Input: part model. Units: mm. Frame: model coordinates. A direction names the side the tool comes from. Give positions to 0.01 mm unless a question says otherwise; leave off trailing zeros. Loops run counter-clockwise (first coordinate to the right, second up) from the corner with the lowest first, then second, coordinate; pieces in that order, holes last. Notation, with made-up numbers: M -24.75,-26.5 L -13.75,-26.5 A11 ccw -13.75,-5.5 Z; hole C 17,-12.5 d5. An arc over 180 degrees is marked long. Use a Markdown table: item, result. Add a question column.
from build123d import *

# Parameters (mm, degrees)
F0_W      = 200
F0_H      = 150
F0_R      = 10
F1_DEPTH  = 100
F2_DEPTH  = 20
F3_W      = 100
F3_H      = 10
F4_DEPTH  = 50
F5_SIZE   = 30
F6_W      = 70
F6_H      = 10
F7_DEPTH  = 130
F8_R      = 4.99999
F9_R      = 10
F10_DEPTH = 20


# Not quite as in the source:
# - a fillet or chamfer is up to 0.001 mm smaller than in the source, because OpenCascade refuses the exact size


with BuildPart() as f1:
    # F0 (on Top) → F1 (new body)
    with BuildSketch(Plane.XY):
        with Locations((-14.7118499619, 7.1657538414)):
            Rectangle(F0_W, F0_H)
        with Locations((-14.7118499619, 7.1657538414)):
            Circle(F0_R, mode=Mode.SUBTRACT)
        with Locations((-14.7118499619, 7.1657538414)):
            Circle(F0_R)
    extrude(amount=F1_DEPTH)

    # F0 (on Top) → F2 (join)
    with BuildSketch(Plane.XY):
        with Locations((-14.7118499619, 7.1657538414)):
            Circle(F0_R)
    extrude(amount=-F2_DEPTH)

    # F3 (on face) → F4 (join)
    with BuildSketch(Plane.XY.offset(100)):
        with Locations((-64.7118499619, 77.1657538414)):
            Rectangle(F3_W, F3_H)
        with Locations((-64.7118499619, -62.8342461586)):
            Rectangle(F3_W, F3_H)
    extrude(amount=F4_DEPTH)

    # F5
    f5_edges = [f1.edges().sort_by_distance(p)[0] for p in [
        (-14.71185, -62.834246, 150),
        (-14.71185, 77.165754, 150),
    ]]
    chamfer(f5_edges, length=F5_SIZE)

    # F6 (on face) → F7 (join)
    with BuildSketch(Plane.XZ.offset(-72.1657538414)):
        with Locations((-79.7118499619, 145)):
            Rectangle(F6_W, F6_H)
        Polygon((-34.7118499619, 140), (-44.7118499619, 150), (-44.7118499619, 140), align=None)
    extrude(amount=F7_DEPTH)

    # F8 (radius 5 in the source; OpenCascade refuses exactly that, so slightly less here)
    f8_edges = [f1.edges().sort_by_distance(p)[0] for p in [
        (35.28815, 82.165754, 100),
        (35.28815, -67.834246, 100),
        (-14.71185, 82.165754, 0),
        (-14.71185, -67.834246, 0),
        (-114.71185, 82.165754, 75),
        (-114.71185, 7.165754, 150),
        (-114.71185, -67.834246, 75),
        (-114.71185, 7.165754, 0),
        (-114.71185, 72.165754, 120),
        (-114.71185, 7.165754, 100),
        (-114.71185, -57.834246, 120),
        (-114.71185, 7.165754, 140),
        (-14.71185, -62.834246, 120),
        (-44.71185, 7.165754, 150),
        (-14.71185, 77.165754, 120),
    ]]
    fillet(f8_edges, radius=F8_R)

    # F9 (on face) → F10 (cut)
    with BuildSketch(Plane.YZ.offset(85.2881500381)):
        with Locations((7.1657538414, 50)):
            Circle(F9_R)
    extrude(amount=-F10_DEPTH, mode=Mode.SUBTRACT)


solid = f1.part
1) Section query C-C, the plane x = 10. Return the cut outline in (y, z).
2) Ray query, line 1 (Z direction, x = -90, y = 30.5); line 2 (Z direction, x = 71.5, y = 60.5); line 3 (X direction, y = 11.5, z = 46). Return the intervals inside material, ascending. Write a range as [from, to].
3) Section query D-D, the plane x = -40.5. Return the cut outline in (y, z).
4) Pull-direction query (Z, two-part tool) for faces 5 (the cylindrical face through (-113.29, 80.66, 76.48)), 6 (the flat face through (-14, 24, 0)), 7 (the flat face through (-73, 8, 140)); classes: pulls with the +Z half, pulls with the -Z half, needs draft (parallel to the pull), parting line crosses it, or undercut.
5) Section query B-B, the plane x = -90.5. Return the cut outline in (y, z), and give its area (3 significant figures).
6) Contact query for flat-ended pins moving along their axis: P1, Ø3, axis at x = -5, y = -21.5, coming from the -Z side; P2, Ø6, axis at y = 9, z = 50, coming from the +X side; P3, Ø11, axis at y = 75, z = 105, coming from the +X side; P4, Ø12, axis at x = -80, z = -2.5, coming from the +Y side. Output: stop coordinate, or through.
7) Reachability of faces 1 (the flat face through (-63, 72.166, 120)), 2 (the cylindrical face through (75.428, 4.998, 40.238)), 3 (the cylindrical face through (-113.286, 6.186, 141.504)), 4 (the cylindrical face through (-16.01, 17.08, -9.86)) from +Z, -Z, +X, -X, +Y, -Y: full face, straight path, thin tool, end or side. Return the list, or none.
Entries:
| question | item | result |
|---|---|---|
| 1 | outline | M -67.83,5 A5 ccw -62.83,0 L 77.17,0 A5 ccw 82.17,5 L 82.17,95 A5 ccw 77.17,100 L -62.83,100 A5 ccw -67.83,95 Z |
| 2 | line 1 | z = [0, 100], [140, 150] |
| 2 | line 2 | z = [0, 100] |
| 2 | line 3 | x = [-114.71, 65.29] |
| 3 | outline | M -67.83,5 A5 ccw -62.83,0 L 77.17,0 A5 ccw 82.17,5 L 82.17,145.79 L -67.83,145.79 Z; hole M -57.83,100 L 72.17,100 L 72.17,140 L -57.83,140 Z |
| 4 | face 5 | needs draft |
| 4 | face 6 | pulls with the -Z half |
| 4 | face 7 | undercut |
| 5 | outline | M -67.83,5 A5 ccw -62.83,0 L 77.17,0 A5 ccw 82.17,5 L 82.17,150 L -67.83,150 Z; hole M -57.83,100 L 72.17,100 L 72.17,140 L -57.83,140 Z |
| 5 | area | 17,300 mm² |
| 6 | P1 | stops at z = 0 |
| 6 | P2 | stops at x = 65.29 |
| 6 | P3 | stops at x = 85.29 |
| 6 | P4 | stops at y = 81.94 |
| 7 | face 1 | +X, -X |
| 7 | face 2 | +X |
| 7 | face 3 | -X |
| 7 | face 4 | -Z |
